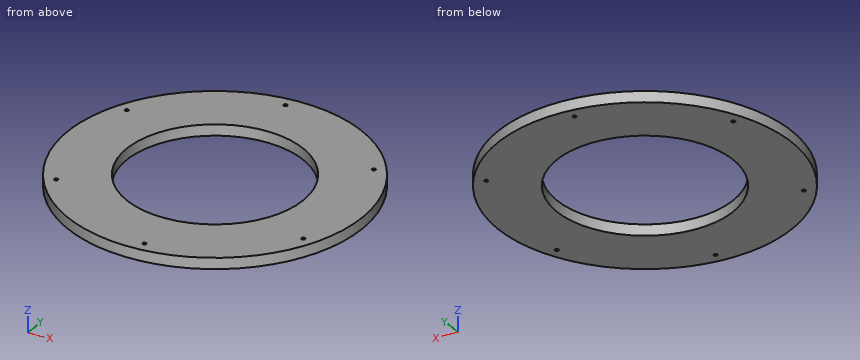
from build123d import *

# Parameters (mm, degrees)
F0_R     = 254
F0_R_2   = 152.4
F1_DEPTH = 19.05


with BuildPart() as f1:
    # F0 (on Top) → F1 (new body)
    with BuildSketch(Plane.XY):
        Circle(F0_R)
        with BuildLine():
            ThreePointArc((196.7011125508, 128.4919251209), (225.1848450649, 67.0319927579), (234.95, 0))
            ThreePointArc((234.95, 0), (229.2479499847, -51.4478369596), (212.4185683948, -100.3984775836))
            ThreePointArc((212.4185683948, -100.3984775836), (213.7303800146, -101.5698688542), (214.2174677682, -103.259766116))
            ThreePointArc((214.2174677682, -103.259766116), (212.7141648851, -105.9590352298), (209.6278276113, -106.1021978612))
            ThreePointArc((209.6278276113, -106.1021978612), (131.1382553066, -194.9468145294), (19.2616521087, -234.1591152572))
            ThreePointArc((19.2616521087, -234.1591152572), (19.2684021583, -234.2784835874), (19.2706532388, -234.3980214226))
            ThreePointArc((19.2706532388, -234.3980214226), (16.1937508526, -237.5715056053), (12.9267150604, -234.5941229821))
            ThreePointArc((12.9267150604, -234.5941229821), (-103.259766116, -211.0424677682), (-193.1569162861, -133.7606376736))
            ThreePointArc((-193.1569162861, -133.7606376736), (-197.5812309419, -132.9103938918), (-196.7011125508, -128.4919251209))
            ThreePointArc((-196.7011125508, -128.4919251209), (-234.3980214226, -16.0956532388), (-212.4185683948, 100.3984775836))
            ThreePointArc((-212.4185683948, 100.3984775836), (-213.8943930083, 104.6551683608), (-209.6278276113, 106.1021978612))
            ThreePointArc((-209.6278276113, 106.1021978612), (-131.1382553066, 194.9468145294), (-19.2616521087, 234.1591152572))
            ThreePointArc((-19.2616521087, 234.1591152572), (-16.3131620664, 237.5655622526), (-12.9267150604, 234.5941229821))
            ThreePointArc((-12.9267150604, 234.5941229821), (103.259766116, 211.0424677682), (193.1569162861, 133.7606376736))
            ThreePointArc((193.1569162861, 133.7606376736), (196.4296661871, 133.9457053883), (198.1218145294, 131.1382553066))
            ThreePointArc((198.1218145294, 131.1382553066), (197.744181257, 129.6364682408), (196.7011125508, 128.4919251209))
        make_face(mode=Mode.SUBTRACT)
        with BuildLine():
            ThreePointArc((212.4185683948, -100.3984775836), (229.2479499847, -51.4478369596), (234.95, 0))
            ThreePointArc((234.95, 0), (225.1848450649, 67.0319927579), (196.7011125508, 128.4919251209))
            ThreePointArc((196.7011125508, 128.4919251209), (192.3123981168, 129.3661167214), (193.1569162861, 133.7606376736))
            ThreePointArc((193.1569162861, 133.7606376736), (103.259766116, 211.0424677682), (-12.9267150604, 234.5941229821))
            ThreePointArc((-12.9267150604, 234.5941229821), (-12.9221690561, 234.4961190364), (-12.9206532388, 234.3980214226))
            ThreePointArc((-12.9206532388, 234.3980214226), (-15.9761154036, 231.2252725031), (-19.2616521087, 234.1591152572))
            ThreePointArc((-19.2616521087, 234.1591152572), (-131.1382553066, 194.9468145294), (-209.6278276113, 106.1021978612))
            ThreePointArc((-209.6278276113, 106.1021978612), (-208.3431986543, 104.931463233), (-207.8674677682, 103.259766116))
            ThreePointArc((-207.8674677682, 103.259766116), (-209.3525705064, 100.5718538695), (-212.4185683948, 100.3984775836))
            ThreePointArc((-212.4185683948, 100.3984775836), (-234.3980214226, -16.0956532388), (-196.7011125508, -128.4919251209))
            ThreePointArc((-196.7011125508, -128.4919251209), (-193.4450274636, -128.3408885789), (-191.7718145294, -131.1382553066))
            ThreePointArc((-191.7718145294, -131.1382553066), (-192.1393644477, -132.6211069643), (-193.1569162861, -133.7606376736))
            ThreePointArc((-193.1569162861, -133.7606376736), (-103.259766116, -211.0424677682), (12.9267150604, -234.5941229821))
            ThreePointArc((12.9267150604, -234.5941229821), (15.8781444113, -231.2304805925), (19.2616521087, -234.1591152572))
            ThreePointArc((19.2616521087, -234.1591152572), (131.1382553066, -194.9468145294), (209.6278276113, -106.1021978612))
            ThreePointArc((209.6278276113, -106.1021978612), (208.190542528, -101.8643638712), (212.4185683948, -100.3984775836))
        make_face()
        Circle(F0_R_2, mode=Mode.SUBTRACT)
    extrude(amount=F1_DEPTH)


solid = f1.part
Could you check a few things on this model? Use its own coordinates, in mm. Coordinates: 2 decimals unless noted, no trailing zeros. Write each loop counter-clockwise with the first axis right and the second up, starting at its lowest first coordinate (ties: lowest second). Pieces come first, ordered by that corner, then holes. Notation, with made-up numbers: (53.5, -11) - (80.5, -11) arc R26 ccw to (80.5, 23) - close; hole circle Ø6 at (84.5, 4). An arc over 180 degrees is marked (long way). Put each result on its own line as item: value. Start each with the question number.
Q1. Please list where these lines run through material, in increasing order: L1, parallel to Y at x = 0, z = 5.5; L2, parallel to Y at x = 102.5, z = 6.75; L3, parallel to X at y = 135, z = 2.
Q2. I want a section at A-A on y = 0. Write out the boundary of the cut face in (x, z).
Q3. I'm going to push flat-ended pins straight in: P1, Ø10, axis at y = -12, z = 6.5, coming from the -X side; P2, Ø8, axis at x = -47, z = 14, coming from the +Y side; P3, Ø1.5, axis at y = 32, z = 15.5, coming from the -X side. Where does each tip first touch, or does it pass through?
Q4. I want a section at C-C on z = 10.25. Write out the boundary of the cut face in (x, y) (3 decimals).
Checks:
1. L1: -254 to -152.4, 152.4 to 254
1. L2: -232.4 to -112.78, 112.78 to 232.4
1. L3: -215.15 to -70.72, 70.72 to 215.15
2. outline: (-254, 0) - (-152.4, 0) - (-152.4, 19.05) - (-254, 19.05) - close; (152.4, 0) - (254, 0) - (254, 19.05) - (152.4, 19.05) - close
3. P1: x = -253.9
3. P2: y = 250.33
3. P3: x = -252.07
4. outline: circle Ø508 at (0, 0); hole circle Ø6.35 at (-211.042, 103.26); hole circle Ø6.35 at (-194.947, -131.138); hole circle Ø304.8 at (0, 0); hole circle Ø6.35 at (-16.096, 234.398); hole circle Ø6.35 at (16.096, -234.398); hole circle Ø6.35 at (194.947, 131.138); hole circle Ø6.35 at (211.042, -103.26)
